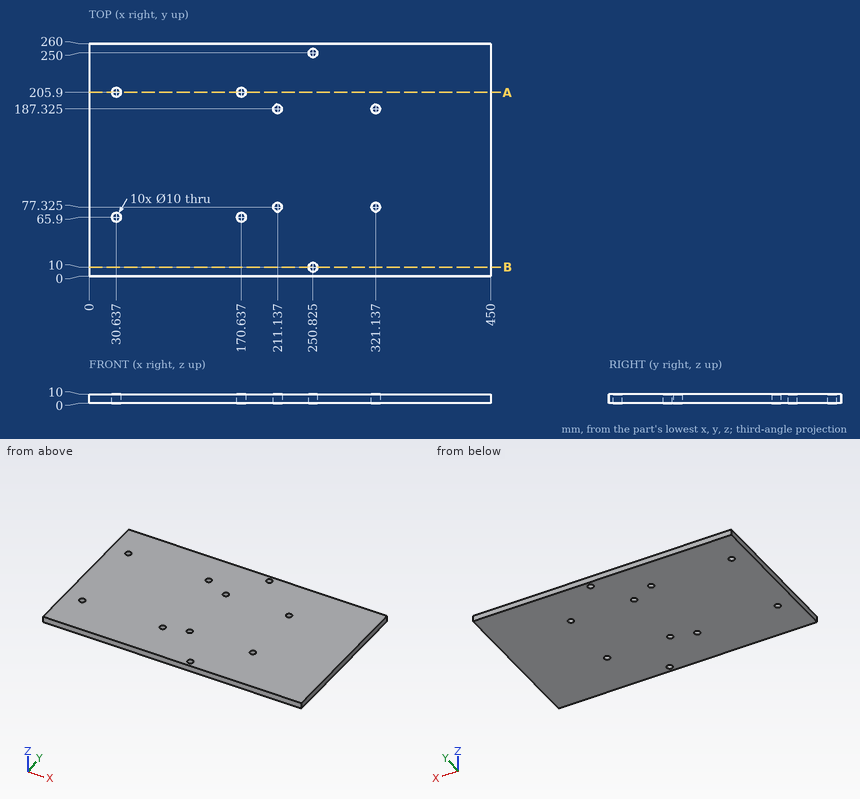
Can you work these out from the drawing? Everything is in mm from the part's minimum corner. Give positions to 0.01 mm unless a question says otherwise; leave off trailing zeros. Loops run counter-clockwise (first coordinate to the right, second up) from the corner with the lowest first, then second, coordinate; pieces in that order, holes last. Notation, with made-up numbers: M 30,-32.5 L 84,-32.5 A22 ccw 84,-8.5 Z; hole C -26,39 d1. An arc over 180 degrees is marked long. Use CSV: the item, a comma, the result in double quotes. Start each with the question number.
1. Imagine slicing it at B-B, the plane y = 10. Write out the boundary of the cut face in (x, z) (1 decimal).
2. Imagine slicing it at A-A, the plane y = 205.9. Write out the boundary of the cut face in (x, z).
3. If I drill on L1, parallel to X at y = 205.9, z = 7.5; L2, parallel to X at y = 10, z = 6.5 (1 decimal); L3, parallel to Y at x = 254.5, z = 9, over which ranges is the centre line in solid material (lowest first)?
Response values:
1,outline,"M 0,0 L 245.8,0 L 245.8,10 L 0,10 Z; M 255.8,0 L 450,0 L 450,10 L 255.8,10 Z"
2,outline,"M 0,0 L 25.64,0 L 25.64,10 L 0,10 Z; M 35.64,0 L 165.64,0 L 165.64,10 L 35.64,10 Z; M 175.64,0 L 450,0 L 450,10 L 175.64,10 Z"
3,L1,"0 to 25.64, 35.64 to 165.64, 175.64 to 450"
3,L2,"0 to 245.8, 255.8 to 450"
3,L3,"0 to 6.61, 13.39 to 246.61, 253.39 to 260"
